Can you work these out from the drawing? Everything is in mm from the part's minimum corner. A direction names the side the tool comes from. Round coordinates to 2 decimals unless told otherwise and drop trailing zeros. Write each loop counter-clockwise with the first axis right and the second up, starting at its lowest first coordinate (ties: lowest second). Pieces come first, ordered by that corner, then holes. Notation, with made-up numbers: (-6.75, 20.5) - (29.25, 20.5) arc R27 ccw to (29.25, 59.5) - close; hole circle Ø8 at (44, -32.75). An arc over 180 degrees is marked (long way). Write each question's results on one line, items separated by ' | '. Start each with the question number.
(1) Imagine slicing it at C-C on z = 13.5. Write out the boundary of the cut face in (x, y).
(2) Please list where these lines run through material, in increasing order: line 1 (Z direction, x = 23, y = 7.75); line 2 (X direction, y = 3.25, z = 6) (1 decimal); line 3 (X direction, y = 8.25, z = 8.5) (1 decimal). Write a range as [from, to].
(3) Imagine slicing it at B-B on x = 33. Write out the boundary of the cut face in (y, z), then the cut area to 3 significant figures.
(4) Imagine slicing it at A-A on y = 6. Write out the boundary of the cut face in (x, z), then the cut area to 3 significant figures.
(5) On a 3-axis mill with a long thin cutter (end or side, diameter ignored), from which of +Z, -Z, +X, -X, +Y, -Y can I reach the whole of each face in a straight line? I mean the marked faces 5 and 6. Say none if no direction works.
(6) Thinking about a two-plate mould opening in X: for the marked faces 1, 2, 3 and 4, which applies, +X half, -X half, draft (parallel to the pull), parting line (faces both ways), or undercut?
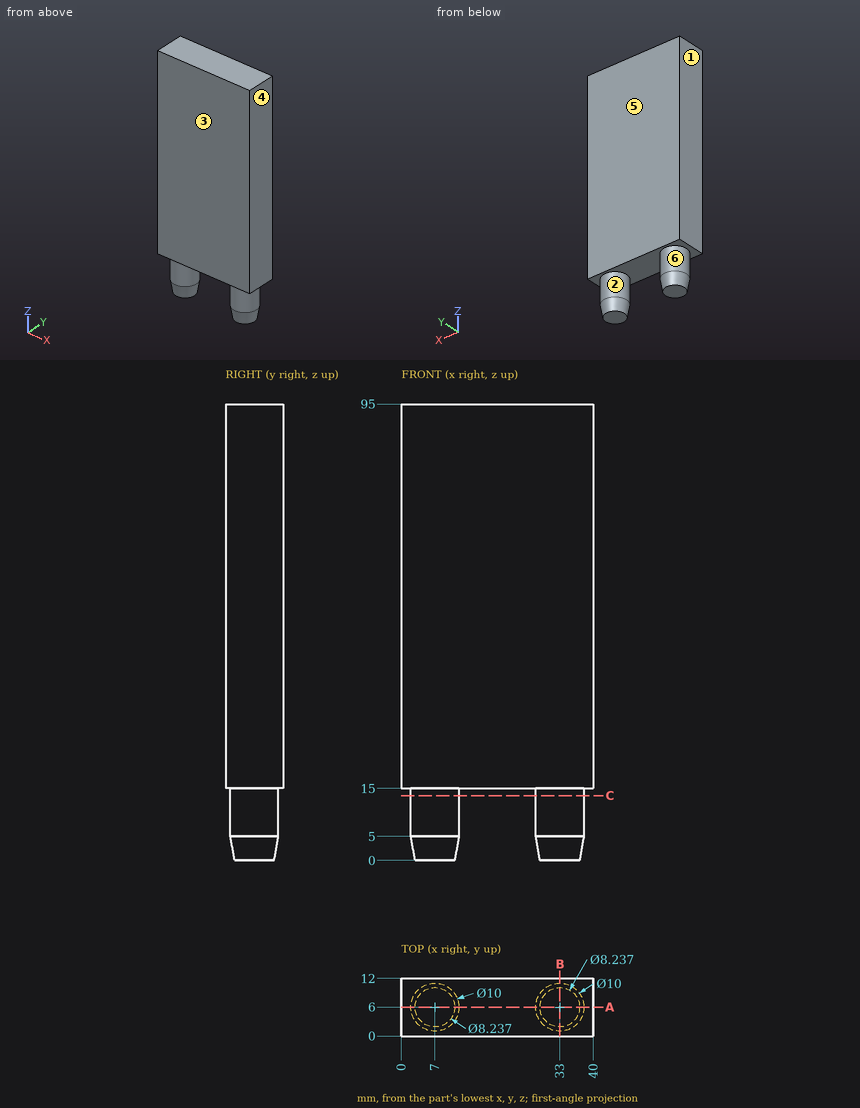
Response:
1) outline: circle Ø10 at (7, 6); circle Ø10 at (33, 6)
2) line 1: [15, 95] | line 2: [2.8, 11.2], [28.8, 37.2] | line 3: [2.5, 11.5], [28.5, 37.5]
3) outline: (0, 15) - (1, 15) - (1, 5) - (1.88, 0) - (10.12, 0) - (11, 5) - (11, 15) - (12, 15) - (12, 95) - (0, 95) - close | area: 1,110 mm²
4) outline: (0, 15) - (2, 15) - (2, 5) - (2.88, 0) - (11.12, 0) - (12, 5) - (12, 15) - (28, 15) - (28, 5) - (28.88, 0) - (37.12, 0) - (38, 5) - (38, 15) - (40, 15) - (40, 95) - (0, 95) - close | area: 3,490 mm²
5) face 5: +Z, -Z, +X, -X, +Y | face 6: -Z
6) face 1: -X half | face 2: undercut | face 3: draft | face 4: +X half
